Can you work these out from the model? Positions are in its coordinate system, mm. A direction names the side the tool comes from. Coordinates: 2 decimals unless noted, no trailing zeros. Order: outer loops, then holes, each group sorted by start corner. A loop starts at its lowest first (then second) coordinate and runs counter-clockwise, first axis right, second up. Notation, with made-up numbers: (-38.75, -2.5) -> (-32.75, -2.5) arc R22 cw to (-32.75, 16.5) -> close; hole circle Ø11 at (47.25, 43). An arc over 180 degrees is marked (long way). Answer in a Markdown table with one row per item.
```python
from build123d import *

# Parameters (mm, degrees)
BOSS_EXTRUDE1_DEPTH = 2
SKETCH2_R           = 1.92051595
SKETCH2_R_2         = 1
CUT_EXTRUDE1_DEPTH  = 10


with BuildPart() as part:
    # Sketch1 → Boss-Extrude1 (new body)
    with BuildSketch(Plane(origin=(0, 0, 0), x_dir=(1, 0, 0), z_dir=(0, 1, 0))):
        Polygon((0, 0), (4.532648702, 0), (6.532648702, -3), (12.5, -3), (16, 1.375958147), (16, 4.543860935), (20, 6.543860935), (20, 44), (16, 46), (16, 56), (9.5, 59), (9.5, 65), (12.5, 67), (12.5, 72), (9.5, 74), (9.5, 80), (12.5, 82), (12.5, 87), (9.5, 89), (9.5, 95), (12.5, 97), (12.5, 100), (9.5, 102), (0, 102), (0, 49), (2.671572875, 49), (4.085786438, 50.414213562), (6.085786438, 50.414213562), (7.5, 49), (7.5, 47), (6.085786438, 45.585786438), (4.085786438, 45.585786438), (2.671572875, 47), (0, 47), (0, 7), (2.671572875, 7), (4.085786438, 8.414213562), (6.085786438, 8.414213562), (7.5, 7), (7.5, 5), (6.085786438, 3.585786438), (4.085786438, 3.585786438), (2.671572875, 5), (0, 5), align=None)
        Polygon((3.111649133, 94.44670143), (5.111649133, 94.44670143), (6.525862696, 93.032487868), (6.525862696, 91.032487868), (5.111649133, 89.618274306), (5.111649133, 84.275128555), (6.525862696, 82.860914993), (6.525862696, 80.860914993), (5.111649133, 79.44670143), (3.111649133, 79.44670143), (1.697435571, 80.860914993), (1.697435571, 82.860914993), (3.111649133, 84.275128555), (3.111649133, 89.618274306), (1.697435571, 91.032487868), (1.697435571, 93.032487868), align=None, mode=Mode.SUBTRACT)
        Polygon((3.111649133, 72.74417146), (5.111649133, 72.74417146), (6.525862696, 71.329957898), (6.525862696, 69.329957898), (5.111649133, 67.915744336), (5.111649133, 62.572598585), (6.525862696, 61.158385023), (6.525862696, 59.158385023), (5.111649133, 57.74417146), (3.111649133, 57.74417146), (1.697435571, 59.158385023), (1.697435571, 61.158385023), (3.111649133, 62.572598585), (3.111649133, 67.915744336), (1.697435571, 69.329957898), (1.697435571, 71.329957898), align=None, mode=Mode.SUBTRACT)
    boss_extrude1 = extrude(amount=BOSS_EXTRUDE1_DEPTH)

    # Mirror1: Boss-Extrude1 across plane
    add(boss_extrude1.mirror(Plane(origin=(0, 0, 0), x_dir=(0, 0, 1), z_dir=(1, 0, 0))))

    # Sketch2 → Cut-Extrude1 (cut)
    with BuildSketch(Plane(origin=(0, 2, 0), x_dir=(1, 0, 0), z_dir=(0, 1, 0))):
        with Locations((-0.199550917, 26.529752726)):
            Circle(SKETCH2_R)
        with Locations((-8.199550917, 34.529752726)):
            Circle(SKETCH2_R_2)
        with Locations((-0.199550917, 34.529752726)):
            Circle(SKETCH2_R_2)
        with Locations((7.800449083, 34.529752726)):
            Circle(SKETCH2_R_2)
        with Locations((7.800449083, 26.529752726)):
            Circle(SKETCH2_R_2)
        with Locations((7.800449083, 18.529752726)):
            Circle(SKETCH2_R_2)
        with Locations((-0.199550917, 18.529752726)):
            Circle(SKETCH2_R_2)
        with Locations((-8.199550917, 18.529752726)):
            Circle(SKETCH2_R_2)
        with Locations((-8.199550917, 26.529752726)):
            Circle(SKETCH2_R_2)
        with Locations((-11.5, 42.089017941)):
            Circle(SKETCH2_R_2)
        with Locations((11.5, 42.089017941)):
            Circle(SKETCH2_R_2)
        with Locations((11.5, 11.285069421)):
            Circle(SKETCH2_R_2)
        with Locations((-11.5, 11.285069421)):
            Circle(SKETCH2_R_2)
    extrude(amount=-CUT_EXTRUDE1_DEPTH, mode=Mode.SUBTRACT)


solid = part.part
```
(1) I need wall thicknesses on line 1 (X direction, y = 1.65, z = -91.5); line 2 (X direction, y = 1.6, z = -63); line 3 (Z direction, x = 11.5, y = 0.7). Which ranges of each line are inside material? Lowest first, please. Write a range as [from, to].
Response values:
| item | result |
|---|---|
| line 1 | [-9.5, -6.53], [-1.7, 1.7], [6.53, 9.5] |
| line 2 | [-9.5, -5.11], [-3.11, 3.11], [5.11, 9.5] |
| line 3 | [-100.67, -96.33], [-87.67, -81.33], [-72.67, -66.33], [-58.08, -43.09], [-41.09, -12.29], [-10.29, 3] |
(2) We'd pull the mould along X, two halves only. Please class faces 4 (the flat face through (0, 1, -5)), 5 (the flat face through (-11, 1, -101)), 6 (the flat face through (12.5, 1, -69)): +X half, -X half, draft (parallel to the pull), parting line (faces both ways), or undercut.
Response values:
| item | result |
|---|---|
| face 4 | undercut |
| face 5 | -X half |
| face 6 | +X half |
(3) Suppose I cut it at B-B (y = 0.9). Count the separate pieces of the cut face and the enclosed holes in it, and give its area (3 significant figures).
Response values:
| item | result |
|---|---|
| separate pieces | 1 |
| enclosed holes | 19 |
| area | 2,820 mm2 |
(4) Suppose I cut it at A-A (x = -11.5). Please give me the cut outline in (y, z).
Response values:
| item | result |
|---|---|
| outline | (0, -100.67) -> (2, -100.67) -> (2, -96.33) -> (0, -96.33) -> close; (0, -87.67) -> (2, -87.67) -> (2, -81.33) -> (0, -81.33) -> close; (0, -72.67) -> (2, -72.67) -> (2, -66.33) -> (0, -66.33) -> close; (0, -58.08) -> (2, -58.08) -> (2, -43.09) -> (0, -43.09) -> close; (0, -41.09) -> (2, -41.09) -> (2, -12.29) -> (0, -12.29) -> close; (0, -10.29) -> (2, -10.29) -> (2, 3) -> (0, 3) -> close |
(5) Will these pins go through, and if not, where does the flat tip stop? pin 1 Ø0.6 at (y, z) = (0.5, -70) entering from -X; pin 2 Ø0.6 at (y, z) = (1, -82) entering from +X; pin 3 Ø3.5 at (x, z) = (-0.2, -26.53) entering from +Y; pin 4 Ø1 at (x, y) = (14, 2) entering from +Z.
Response values:
| item | result |
|---|---|
| pin 1 | x = -12.5 |
| pin 2 | x = 12.5 |
| pin 3 | through |
| pin 4 | z = 1.75 |
(6) On a 3-axis mill with a long thin cutter (end or side, diameter ignored), from which of +Z, -Z, +X, -X, +Y, -Y can I reach the whole of each face in a straight line? I mean faces 1 (the flat face through (-11, 1, -88)), 2 (the flat face through (11, 1, -81)), 3 (the flat face through (4, 1, -57.744)). Say none if no direction works.
Response values:
| item | result |
|---|---|
| face 1 | -X, +Y, -Y |
| face 2 | +X, +Y, -Y |
| face 3 | +Y, -Y |
